Autodesk Inventor part; units mm, degrees
ref_plane "YZ Plane" through (0, 0, 0) normal (1, 0, 0) x (0, 1, 0)
ref_plane "XZ Plane" through (0, 0, 0) normal (0, 1, 0) x (-1, 0, 0)
ref_plane "XY Plane" through (0, 0, 0) normal (0, 0, 1) x (1, 0, 0)
sketch "Sketch1" plane through (0, 0, 0) normal (0, 1, 0) x (-1, 0, 0)
  line L0 (0, 0) -> (0, -15.8369)
  line L1 (0, -15.8369) -> (15.8369, -15.8369)
  line L2 (15.8369, -15.8369) -> (15.8369, 0)
  line L3 (15.8369, 0) -> (0, 0)
  dimension "d0" = 15.8369
  dimension "d1" = 15.8369
  dimension "d2" = 15.8369
extrude "Extrusion1" add sketch "Sketch1" along normal blind 3.236
sketch "Sketch2" plane through (0, 3.236, 0) normal (0, 1, 0) x (1, 0, 0)
  line L0 (-15.8369, 15.8369) -> (-15.8369, 0)
  line L1 (-15.8369, 0) -> (0, 15.8369)
  line L2 (0, 15.8369) -> (-15.8369, 15.8369)
  line L3 (-15.8369, 15.8369) -> (0, 0)
  line L4 (-7.9185, 7.9185) -> (0, 7.9185)
  line L5 (0, 7.9185) -> (-15.8369, 7.9185)
  line L6 (-7.9185, 7.9185) -> (-7.9185, 15.8369)
  line L7 (0, 15.8369) -> (-15.8369, 15.8369)
  line L8 (-7.9185, 0) -> (-7.9185, 7.9185)
  line L9 (-7.9185, 0) -> (-15.8369, 7.9185)
  line L10 (-15.8369, 7.9185) -> (-7.9185, 15.8369)
  line L11 (0, 7.9185) -> (-7.9185, 15.8369)
  line L12 (-7.9185, 0) -> (0, 7.9185)
  circle A0 centre (-11.8777, 3.9592) radius 2.4498
  dimension "d5" = 4.8997
extrude "Extrusion2" add sketch "Sketch2" along normal blind 1.9837 contours A0 L1 L9 | L9 L1 A0 | L1 L9 A0 | A0 L9 L1
pattern_linear "Rectangular Pattern1" count 2 spacing 7.7978 along (1, 0, 0) count 2 spacing 7.7978 along (0, 0, -1) of "Extrusion2"
shell "Shell1" thickness 1.4732 removed faces 1 at (-5.279, 0, -10.5579)
sketch "Sketch3" plane through (0, 0, 0) normal (0, 1, 0) x (-1, 0, 0)
  circle A0 centre (4.0799, -3.9592) radius 2.4498 construction
  circle A1 centre (11.8777, -11.757) radius 2.4498 construction
  line L0 (4.0799, -3.9592) -> (11.8777, -11.757) construction
  circle A2 centre (7.9788, -7.8581) radius 3.064
  circle A3 centre (7.9788, -7.8581) radius 2.4498
  point P0 (0, 0)
  dimension "d15" = 4.8997
extrude "Extrusion3" add sketch "Sketch3" along normal up to surface (1.7628 mm away)
properties part number "2x2 short orange pegged" material "ABS Plastic"
The listing builds one solid part. Answer for the finished solid, in the listing's coordinates (mm). A direction names the side the tool comes from. Coordinates: 2 decimals unless noted, no trailing zeros. Order: outer loops, then holes, each group sorted by start corner. A loop starts at its lowest first (then second) coordinate and runs counter-clockwise, first axis right, second up. Notation, with made-up numbers: (66, -24.75) -> (117, -24.75) arc R20 cw to (117, -10.75) -> close; hole circle Ø4 at (87, 85.5). An arc over 180 degrees is marked (long way). Answer in a Markdown table with one row per item. Add a question column.
Item 1: Find section C-C (x = -14). Write down the section's boundary in (y, z).
Item 2: Find section B-B (y = 3.55). Write down the section's boundary in (x, z).
Item 3: Determine the mould class of faces 4 (the face through (-15.837, 2, -8)), 5 (the face through (-8, 2, 0)), 6 (the face through (-14.364, 1, -8)) for opening direction X: +X half, -X half, draft (parallel to the pull), parting line (faces both ways), or undercut.
Item 4: Find section A-A (y = 1.3). Write down the section's boundary in (x, z), then the cut area to 3 significant figures.
Item 5: Find section D-D (z = -13.5). Write down the section's boundary in (x, y), then the cut area to 3 significant figures.
Item 6: Which of the six approach directions +Z, -Z, +X, -X, +Y, -Y give full straight-line access (tool end or side, diameter ignored) to faces 1 (the face through (-10.9, 0.87, -8.78)), 2 (the face through (-1.82, 4.21, -12.7)), 3 (the face through (-8, 2, -15.837))?
Item 7: Find the intervals of material crossed by L1, parallel to X at y = 2.4, z = -4; L2, parallel to Z at x = -11.75, y = 4.2; L3, parallel to X at y = 1.25, z = -14, in increasing order. Write a range as from..to.
Item 8: Each of these flat-tipped pins is pushed along its axis until it touches: P1, Ø0.6, axis at x = -12, z = -3.5, coming from the -Y side; P2, Ø4, axis at x = -7.98, z = -7.86, coming from the +Y side; P3, Ø1.5, axis at x = -8, z = -8.5, coming from the -Y side. Where does it stop, or does it pass through?
Result set:
| question | item | result |
|---|---|---|
| 1 | outline | (0, -15.84) -> (3.24, -15.84) -> (3.24, -12.98) -> (5.22, -12.98) -> (5.22, -10.53) -> (3.24, -10.53) -> (3.24, -5.18) -> (5.22, -5.18) -> (5.22, -2.74) -> (3.24, -2.74) -> (3.24, 0) -> (0, 0) -> (0, -1.47) -> (1.76, -1.47) -> (1.76, -14.36) -> (0, -14.36) -> close |
| 2 | outline | circle Ø4.9 at (-11.88, -11.76); circle Ø4.9 at (-11.88, -3.96); circle Ø4.9 at (-4.08, -11.76); circle Ø4.9 at (-4.08, -3.96); hole circle Ø1.95 at (-11.88, -11.76); hole circle Ø1.95 at (-11.88, -3.96); hole circle Ø1.95 at (-4.08, -11.76); hole circle Ø1.95 at (-4.08, -3.96) |
| 3 | face 4 | -X half |
| 3 | face 5 | draft |
| 3 | face 6 | undercut |
| 4 | outline | (-15.84, -15.84) -> (0, -15.84) -> (0, 0) -> (-15.84, 0) -> close; circle Ø6.13 at (-7.98, -7.86); hole (-14.36, -14.36) -> (-1.47, -14.36) -> (-1.47, -1.47) -> (-14.36, -1.47) -> close; hole circle Ø4.9 at (-7.98, -7.86) |
| 4 | area | 95.3 mm² |
| 5 | outline | (-15.84, 0) -> (-14.36, 0) -> (-14.36, 1.76) -> (-1.47, 1.76) -> (-1.47, 0) -> (0, 0) -> (0, 3.24) -> (-2.36, 3.24) -> (-2.36, 5.22) -> (-5.8, 5.22) -> (-5.8, 3.24) -> (-10.16, 3.24) -> (-10.16, 5.22) -> (-13.6, 5.22) -> (-13.6, 3.24) -> (-15.84, 3.24) -> close |
| 5 | area | 42.2 mm² |
| 6 | face 1 | -Y |
| 6 | face 2 | +Y |
| 6 | face 3 | -Z, +X, -X, +Y, -Y |
| 7 | L1 | x = -15.84..-12.85, -10.9..-5.06, -3.1..0 |
| 7 | L2 | z = -14.2..-9.31, -6.41..-1.51 |
| 7 | L3 | x = -15.84..-14.36, -1.47..0 |
| 8 | P1 | stops at y = 3.75 |
| 8 | P2 | stops at y = 3.24 |
| 8 | P3 | stops at y = 1.76 |
